```python
from build123d import *

# Parameters (mm, degrees)
EXTRUDE1_DEPTH = 2
SKETCH3_W      = 6
SKETCH3_H      = 6
SKETCH3_R      = 1.5
EXTRUDE2_DEPTH = 2
CHAMFER2_SIZE  = 5


with BuildPart() as part:
    # Sketch1 → Extrude1 (new body)
    with BuildSketch(Plane(origin=(0, 0, 0), x_dir=(1, 0, 0), z_dir=(0, 1, 0))):
        Polygon((-75, 35), (75, 35), (75, -29), (46, -65), (-46, -65), (-75, -29), align=None)
    extrude(amount=EXTRUDE1_DEPTH)

    # Sketch3 → Extrude2 (add)
    # profile 1 of 2: a face of its own
    with BuildSketch(Plane(origin=(0, 2, 0), x_dir=(1, 0, 0), z_dir=(0, 1, 0))):
        with Locations((78, 3)):
            Rectangle(SKETCH3_W, SKETCH3_H)
        with Locations(Location((78, 3, 0), (0, 0, 270))):
            Circle(SKETCH3_R, mode=Mode.SUBTRACT)
    # profile 2 of 2: a face of its own
    with BuildSketch(Plane(origin=(0, 2, 0), x_dir=(1, 0, 0), z_dir=(0, 1, 0))):
        with BuildLine():
            Line((74.824710663, -38.781951728), (70.152187208, -35.0179745))
            Line((70.152187208, -35.0179745), (68.482047894, -37.09125089))
            ThreePointArc((68.482047894, -37.09125089), (70.09994245, -36.822977113), (70.99646032, -38.19622484))
            ThreePointArc((70.99646032, -38.19622484), (69.104945526, -39.644229041), (68.200838766, -37.440338084))
            Line((68.200838766, -37.440338084), (66.388209981, -39.690497955))
            Line((66.388209981, -39.690497955), (71.060733435, -43.454475182))
            Line((71.060733435, -43.454475182), (74.824710663, -38.781951728))
        make_face()
    extrude2 = extrude(amount=-EXTRUDE2_DEPTH)

    # Chamfer2
    chamfer2_edges = [part.edges().sort_by_distance(p)[0] for p in [
        (-75, 1, -35),
        (75, 1, -35),
    ]]
    chamfer(chamfer2_edges, length=CHAMFER2_SIZE)

    # Mirror1: Extrude2 across plane
    add(extrude2.mirror(Plane(origin=(0, 0, 0), x_dir=(0, 0, 1), z_dir=(1, 0, 0))))


solid = part.part
```
Input: part model. Units: mm. Frame: model coordinates. A direction names the side the tool comes from. Coordinates: 2 decimals unless noted, no trailing zeros. Loops run counter-clockwise (first coordinate to the right, second up) from the corner with the lowest first, then second, coordinate; pieces in that order, holes last. Notation, with made-up numbers: M -4.75,-27.5 L 10.25,-27.5 A19 ccw 10.25,5.5 Z; hole C 61.25,-40 d1. An arc over 180 degrees is marked long. One line per item, written item: value.
(1) Section B-B (z = 10.5). Output: boundary loops of the cut face in (x, y), and give its area (3 significant figures).
Filled in:
outline: M -75,0 L 75,0 L 75,2 L -75,2 Z
area: 300 mm^2
(2) Pin query (flat end, axial travel): pin 1 (0.6 mm diameter, centred on y = 0.5, z = 16, fed in from +X); pin 2 (1 mm diameter, centred on x = -77, y = 1, fed in from -Z); pin 3 (1 mm diameter, centred on y = 1, z = 13.5, fed in from -X). Return the tip coordinate at first contact, or that it passes through.
Filled in:
pin 1: x = 75
pin 2: z = -6
pin 3: x = -75
(3) Section C-C (x = 62). Output: boundary loops of the cut face in (y, z).
Filled in:
outline: M 0,-35 L 2,-35 L 2,45.14 L 0,45.14 Z
(4) Reachability of faces 1 (the flat face through (-68.692, 1.014, 41.546)), 2 (the flat face through (-72.542, 0.986, 32.051)), 3 (the flat face through (72.61, 0.99, 31.97)), 4 (the flat face through (-73, 1, -32)), 5 (the cylindrical face through (-79.265, 1.014, -2.194)) from +Z, -Z, +X, -X, +Y, -Y: full face, straight path, thin tool, end or side. Return the list, or none.
Filled in:
face 1: +Z, +Y, -Y
face 2: -X, +Y, -Y
face 3: +X, +Y, -Y
face 4: -Z, -X, +Y, -Y
face 5: +Y, -Y
(5) Line query: line 1 along X through (y, z) = (1.4, -3); line 2 along Z through (x, y) = (-78, 1.2); line 3 along X through (y, z) = (0.25, 29). Output: solid intervals per line, ascending. Write a range as from..to.
Filled in:
line 1: -81..-79.5, -76.5..76.5, 79.5..81
line 2: -6..-4.5, -1.5..0
line 3: -75..75
(6) Section A-A (y = 0.4). Give the number of separate pieces and of enclosed holes in the cut face, and give its area (3 significant figures).
Filled in:
separate pieces: 1
enclosed holes: 4
area: 14,000 mm^2
(7) Pull-direction query (Z, two-part tool) for faces 6 (the flat face through (56.337, 0.986, 52.168)), 7 (the flat face through (1, 2, 14)), 8 (the flat face through (72.521, 1.014, 36.926)), 9 (the flat face through (73, 1, -32)); classes: +Z half, -Z half, draft (parallel to the pull), parting line (faces both ways), or undercut.
Filled in:
face 6: +Z half
face 7: draft
face 8: undercut
face 9: -Z half
